from build123d import *

# Parameters (mm, degrees)
F1_DEPTH     = 10
F2_R         = 4.99999
F3_W         = 7.5
F3_H         = 5
F3_W_2       = 10
F4_DEPTH     = 25.2
F5_T1_DEPTH  = 12
F5_T6_DEPTH  = 10
F5_T11_DEPTH = 10
F5_T17_DEPTH = 29.2876224097
F5_T23_DEPTH = 31.2876224097
F5_T31_DEPTH = 29.2876224097
F5_T37_DEPTH = 31.2876224097
F5_T45_DEPTH = 29.2876224097
F5_T51_DEPTH = 31.2876224097
F5_T59_DEPTH = 31.2876224097
F5_T64_DEPTH = 29.2876224097
F6_R         = 1.5
F7_DEPTH     = 25


# Not quite as in the source:
# - a fillet or chamfer that OpenCascade refuses, or shapes differently, is made with other operations: its cross-section is extruded or revolved along the edge and cut away or added
# - a fillet or chamfer is up to 0.001 mm smaller than in the source, because OpenCascade refuses the exact size


with BuildPart() as f1:
    # F0 (on Front) → F1 (new body)
    with BuildSketch(Plane.XZ):
        Polygon((12.5, -2.5), (12.5, 2.5), (6, 2.5), (-6, 2.5), (-12.5, 2.5), (-12.5, -2.5), align=None)
        Polygon((-6, 2.5), (6, 2.5), (6, 10), (6, 20), (3.5, 20), (3.5, 10), (1.25, 10), (1.25, 20), (0, 20), (-1.25, 20), (-1.25, 10), (-3.5, 10), (-3.5, 20), (-6, 20), (-6, 10), align=None)
    extrude(amount=F1_DEPTH)

    # F2 (radius 5 in the source; OpenCascade refuses exactly that, so slightly less here)
    f2_edges = [f1.edges().sort_by_distance(p)[0] for p in [
        (-4.75, 0, 20),
        (0, 0, 20),
        (4.75, 0, 20),
        (-4.75, -10, 20),
        (0, -10, 20),
        (4.75, -10, 20),
    ]]
    fillet(f2_edges, radius=F2_R)

    # F3 (on face) → F4 (join)
    with BuildSketch(Plane.YZ.offset(12.5)):
        with Locations((-13.75, 0)):
            Rectangle(F3_W, F3_H)
        with Locations((3.75, 0)):
            Rectangle(F3_W, F3_H)
        with Locations((-5, 0)):
            Rectangle(F3_W_2, F3_H)
    extrude(amount=-F4_DEPTH)

    # F5: chamfer of 7.5 on 4 edges, made by hand

    # F5_s2 → F5_t1 (join)
    with BuildSketch(Plane.YZ.offset(-6)):
        Polygon((-17.5, 2.5), (-10, 10), (-10, 2.5), align=None)
        Polygon((7.5, 2.5), (0, 10), (0, 2.5), align=None)
    extrude(amount=F5_T1_DEPTH)


with BuildPart() as f5_tool4:
    # F5_s5 → F5_t6 (new body)
    with BuildSketch(Plane.XZ):
        Polygon((6, 10), (13.5, 2.5), (6, 2.5), align=None)
    extrude(amount=F5_T6_DEPTH)

    split(bisect_by=Plane.YZ.offset(12.5), keep=Keep.BOTTOM)


with BuildPart() as f1_1:
    add(f1.part)

    # F5_t3: union F5_tool4
    add(f5_tool4.part)


with BuildPart() as f5_tool9:
    # F5_s10 → F5_t11 (new body)
    with BuildSketch(Plane.XZ):
        Polygon((-13.5, 2.5), (-6, 10), (-6, 2.5), align=None)
    extrude(amount=F5_T11_DEPTH)

    split(bisect_by=Plane.YZ.offset(-12.7), keep=Keep.TOP)


with BuildPart() as f1_2:
    add(f1_1.part)

    # F5_t8: union F5_tool9
    add(f5_tool9.part)


with BuildPart() as f5_tool15:
    # F5_s16 → F5_t17 (new body)
    with BuildSketch(Plane.XZ):
        Polygon((6, 10), (13.5, 2.5), (6, 2.5), align=None)
    extrude(amount=F5_T17_DEPTH)

    split(bisect_by=Plane.XZ.offset(17.5), keep=Keep.BOTTOM)

    split(bisect_by=Plane.YZ.offset(12.5), keep=Keep.BOTTOM)

    split(bisect_by=Plane.XZ.offset(10), keep=Keep.TOP)


with BuildPart() as f5_tool21:
    # F5_s22 → F5_t23 (new body)
    with BuildSketch(Plane.YZ.offset(25.2876224097)):
        Polygon((-17.5, 2.5), (-10, 10), (-10, 2.5), align=None)
    extrude(amount=-F5_T23_DEPTH)

    split(bisect_by=Plane.YZ.offset(6), keep=Keep.TOP)

    split(bisect_by=Plane.YZ.offset(12.5), keep=Keep.BOTTOM)


with BuildPart() as f5_tool15_1:
    add(f5_tool15.part)

    # F5_t26: intersect F5_tool21
    add(f5_tool21.part, mode=Mode.INTERSECT)


with BuildPart() as f1_3:
    add(f1_2.part)

    # F5_t13: union F5_tool15
    add(f5_tool15_1.part)


with BuildPart() as f5_tool29:
    # F5_s30 → F5_t31 (new body)
    with BuildSketch(Plane.XZ):
        Polygon((-13.5, 2.5), (-6, 10), (-6, 2.5), align=None)
    extrude(amount=F5_T31_DEPTH)

    split(bisect_by=Plane.YZ.offset(-12.7), keep=Keep.TOP)

    split(bisect_by=Plane.XZ.offset(17.5), keep=Keep.BOTTOM)

    split(bisect_by=Plane.XZ.offset(10), keep=Keep.TOP)


with BuildPart() as f5_tool35:
    # F5_s36 → F5_t37 (new body)
    with BuildSketch(Plane.YZ.offset(6)):
        Polygon((-17.5, 2.5), (-10, 10), (-10, 2.5), align=None)
    extrude(amount=-F5_T37_DEPTH)

    split(bisect_by=Plane.YZ.offset(-6), keep=Keep.BOTTOM)

    split(bisect_by=Plane.YZ.offset(-12.7), keep=Keep.TOP)


with BuildPart() as f5_tool29_1:
    add(f5_tool29.part)

    # F5_t40: intersect F5_tool35
    add(f5_tool35.part, mode=Mode.INTERSECT)


with BuildPart() as f1_4:
    add(f1_3.part)

    # F5_t27: union F5_tool29
    add(f5_tool29_1.part)


with BuildPart() as f5_tool43:
    # F5_s44 → F5_t45 (new body)
    with BuildSketch(Plane.XZ.offset(-19.2876224097)):
        Polygon((6, 10), (13.5, 2.5), (6, 2.5), align=None)
    extrude(amount=F5_T45_DEPTH)

    split(bisect_by=Plane.XZ.offset(-7.5), keep=Keep.TOP)

    split(bisect_by=Plane.YZ.offset(12.5), keep=Keep.BOTTOM)

    split(bisect_by=Plane.XZ, keep=Keep.BOTTOM)


with BuildPart() as f5_tool49:
    # F5_s50 → F5_t51 (new body)
    with BuildSketch(Plane.YZ.offset(25.2876224097)):
        Polygon((7.5, 2.5), (0, 10), (0, 2.5), align=None)
    extrude(amount=-F5_T51_DEPTH)

    split(bisect_by=Plane.YZ.offset(6), keep=Keep.TOP)

    split(bisect_by=Plane.YZ.offset(12.5), keep=Keep.BOTTOM)


with BuildPart() as f5_tool43_1:
    add(f5_tool43.part)

    # F5_t54: intersect F5_tool49
    add(f5_tool49.part, mode=Mode.INTERSECT)


with BuildPart() as f1_5:
    add(f1_4.part)

    # F5_t41: union F5_tool43
    add(f5_tool43_1.part)


with BuildPart() as f5_tool57:
    # F5_s58 → F5_t59 (new body)
    with BuildSketch(Plane.YZ.offset(6)):
        Polygon((7.5, 2.5), (0, 10), (0, 2.5), align=None)
    extrude(amount=-F5_T59_DEPTH)

    split(bisect_by=Plane.YZ.offset(-6), keep=Keep.BOTTOM)

    split(bisect_by=Plane.YZ.offset(-12.7), keep=Keep.TOP)


with BuildPart() as f5_tool62:
    # F5_s63 → F5_t64 (new body)
    with BuildSketch(Plane.XZ.offset(-19.2876224097)):
        Polygon((-13.5, 2.5), (-6, 10), (-6, 2.5), align=None)
    extrude(amount=F5_T64_DEPTH)

    split(bisect_by=Plane.XZ.offset(-7.5), keep=Keep.TOP)

    split(bisect_by=Plane.YZ.offset(-12.7), keep=Keep.TOP)

    split(bisect_by=Plane.XZ, keep=Keep.BOTTOM)


with BuildPart() as f5_tool57_1:
    add(f5_tool57.part)

    # F5_t68: intersect F5_tool62
    add(f5_tool62.part, mode=Mode.INTERSECT)


with BuildPart() as f1_6:
    add(f1_5.part)

    # F5_t55: union F5_tool57
    add(f5_tool57_1.part)

    # F6 (on face) → F7 (cut)
    with BuildSketch(Plane(origin=(-6, 0, 0), x_dir=(0, -1, 0), z_dir=(-1, 0, 0))):
        with Locations((5, 16)):
            Circle(F6_R)
    extrude(amount=-F7_DEPTH, mode=Mode.SUBTRACT)


solid = f1_6.part
Input: part model. Units: mm. Frame: model coordinates. A direction names the side the tool comes from. Coordinates: 2 decimals unless noted, no trailing zeros. Order: outer loops, then holes, each group sorted by start corner. A loop starts at its lowest first (then second) coordinate and runs counter-clockwise, first axis right, second up.
1. Access query for faces 1 (the flat face through (6, -5, 14)), 2 (the flat face through (-2, -5, 10)), 3 (the flat face through (5, 0, 13)), 4 (the cylindrical face through (4.732, -6.386, 15.425)), 5 (the flat face through (0, -10, 13)). Directions: +Z, -Z, +X, -X, +Y, -Y. A direction counts if a zero-diameter tool reaches every point of the face in a straight line with its end or side. Return the directions, or none.
Checked values:
face 1: +Z, +X, +Y, -Y
face 2: +Z, +Y, -Y
face 3: +Z, +X, -X, +Y
face 4: +X, -X
face 5: +Z, +X, -X, -Y
2. Cut plane D-D, the plane z = 18.5. Return loops of the section in (x, y).
Checked values:
outline: (-6, -8.57) - (-3.5, -8.57) - (-3.5, -1.43) - (-6, -1.43) - close; (-1.25, -8.57) - (1.25, -8.57) - (1.25, -1.43) - (-1.25, -1.43) - close; (3.5, -8.57) - (6, -8.57) - (6, -1.43) - (3.5, -1.43) - close
3. Cut plane B-B, the plane z = 16. Return loops of the section in (x, y).
Checked values:
outline: (-6, -9.9) - (-3.5, -9.9) - (-3.5, -6.5) - (-6, -6.5) - close; (-6, -3.5) - (-3.5, -3.5) - (-3.5, -0.1) - (-6, -0.1) - close; (-1.25, -9.9) - (1.25, -9.9) - (1.25, -6.5) - (-1.25, -6.5) - close; (-1.25, -3.5) - (1.25, -3.5) - (1.25, -0.1) - (-1.25, -0.1) - close; (3.5, -9.9) - (6, -9.9) - (6, -6.5) - (3.5, -6.5) - close; (3.5, -3.5) - (6, -3.5) - (6, -0.1) - (3.5, -0.1) - close
4. Cut plane C-C, the plane y = -9. Return loops of the section in (x, z), plus the area to 3 significant figures.
Checked values:
outline: (-12.7, -2.5) - (12.5, -2.5) - (12.5, 3.5) - (6, 10) - (6, 18) - (3.5, 18) - (3.5, 10) - (1.25, 10) - (1.25, 18) - (-1.25, 18) - (-1.25, 10) - (-3.5, 10) - (-3.5, 18) - (-6, 18) - (-6, 10) - (-12.7, 3.3) - close
area: 331 mm2
5. Contact query for flat-ended pins moving along their axis: P1, Ø11, axis at y = -4.5, z = 17, coming from the -X side; P2, Ø2, axis at x = -5, z = 12, coming from the +Y side; P3, Ø0.8, axis at x = -4, z = 12, coming from the -Y side. Output: stop coordinate, or through.
Checked values:
P1: stops at x = -6
P2: stops at y = 0
P3: stops at y = -10
6. Cut plane A-A, the plane y = -4. Return loops of the section in (x, z).
Checked values:
outline: (-12.7, -2.5) - (12.5, -2.5) - (12.5, 3.5) - (6, 10) - (6, 14.88) - (3.5, 14.88) - (3.5, 10) - (1.25, 10) - (1.25, 14.88) - (-1.25, 14.88) - (-1.25, 10) - (-3.5, 10) - (-3.5, 14.88) - (-6, 14.88) - (-6, 10) - (-12.7, 3.3) - close; (-6, 17.12) - (-3.5, 17.12) - (-3.5, 19.9) - (-6, 19.9) - close; (-1.25, 17.12) - (1.25, 17.12) - (1.25, 19.9) - (-1.25, 19.9) - close; (3.5, 17.12) - (6, 17.12) - (6, 19.9) - (3.5, 19.9) - close
7. Draft query along X for faces 6 (the flat face through (1.25, -5, 14)), 7 (the flat face through (-12.7, -5, 0)), 8 (the flat face through (0, -17.5, 0)), 9 (the flat face through (-1.25, -5, 14)). Return one class per face: +X half, -X half, draft (parallel to the pull), parting line (faces both ways), or undercut.
Checked values:
face 6: undercut
face 7: -X half
face 8: draft
face 9: undercut
8. Ray query, line 1 along Z through (x, y) = (4.7, -5); line 2 along X through (y, z) = (-2.5, 17.5); line 3 along Z through (x, y) = (1, -7.25). Return the intervals inside material, ascending.
Checked values:
line 1: z = -2.5 to 14.5, 17.5 to 20
line 2: x = -6 to -3.5, -1.25 to 1.25, 3.5 to 6
line 3: z = -2.5 to 19.47
